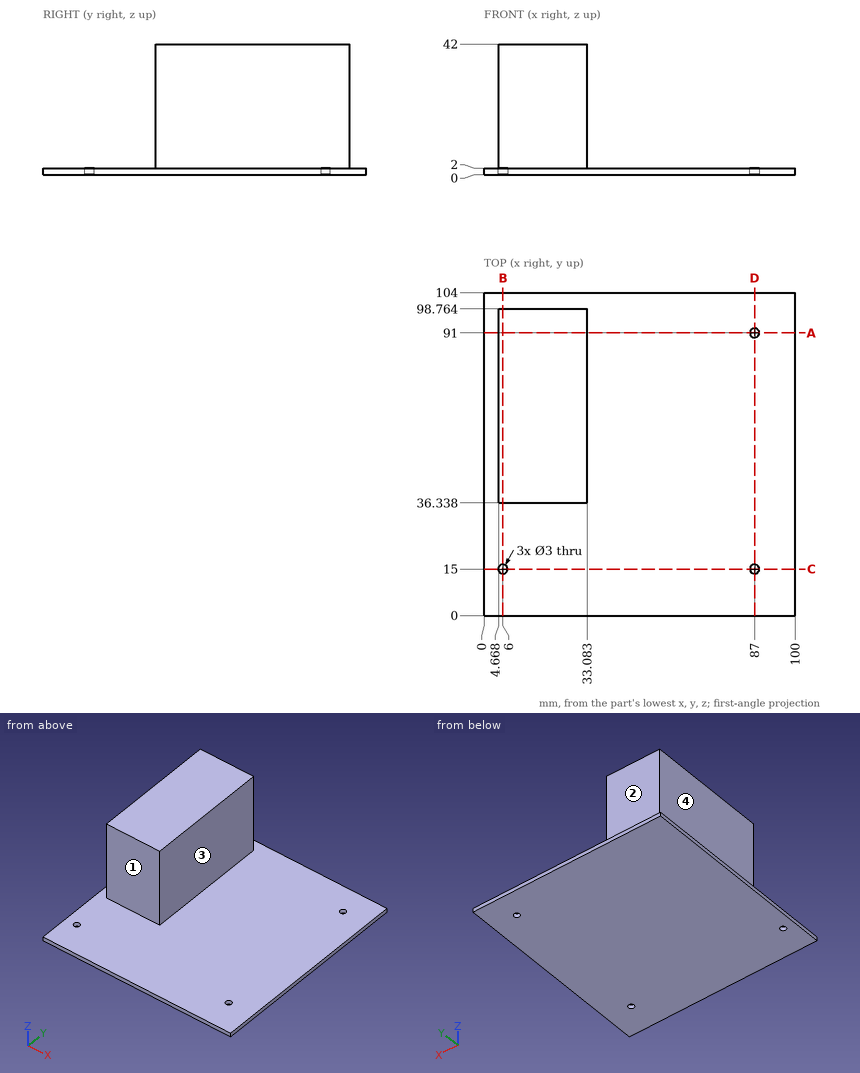
Answer from the drawing. Dimensions are ordinates in mm from the lowest x, y and z of the part. A direction names the side the tool comes from. Coordinates: 2 decimals unless noted, no trailing zeros. Loops run counter-clockwise (first coordinate to the right, second up) from the corner with the lowest first, then second, coordinate; pieces in that order, holes last. Notation, with made-up numbers: (-22, 71.5) -> (29, 71.5) arc R13 cw to (29, 91.5) -> close; hole circle Ø4 at (52.25, 84.25). An arc over 180 degrees is marked (long way). Return JSON: item names as keys, results as strings.
Item 1: For the marked faces 1, 2, 3 and 4, determine the directions among +Z, -Z, +X, -X, +Y, -Y from which every point of the face is accessible in a straight line to the end or side of a thin tool.
Answers:
{"face 1": "+Z, +X, -X, -Y", "face 2": "+Z, +X, -X, +Y", "face 3": "+Z, +X, +Y, -Y", "face 4": "+Z, -X, +Y, -Y"}
Item 2: Find section B-B (x = 6). Determine the outline of the cut face in (y, z).
Answers:
{"outline": "(0, 0) -> (13.5, 0) -> (13.5, 2) -> (0, 2) -> close; (16.5, 0) -> (104, 0) -> (104, 2) -> (98.76, 2) -> (98.76, 42) -> (36.34, 42) -> (36.34, 2) -> (16.5, 2) -> close"}
Item 3: Find section A-A (y = 91). Determine the outline of the cut face in (x, z), plus the area to 3 significant figures.
Answers:
{"outline": "(0, 0) -> (85.5, 0) -> (85.5, 2) -> (33.08, 2) -> (33.08, 42) -> (4.67, 42) -> (4.67, 2) -> (0, 2) -> close; (88.5, 0) -> (100, 0) -> (100, 2) -> (88.5, 2) -> close", "area": "1,330 mm2"}
Item 4: Find section C-C (y = 15). Determine the outline of the cut face in (x, z), plus the area to 3 significant figures.
Answers:
{"outline": "(0, 0) -> (4.5, 0) -> (4.5, 2) -> (0, 2) -> close; (7.5, 0) -> (85.5, 0) -> (85.5, 2) -> (7.5, 2) -> close; (88.5, 0) -> (100, 0) -> (100, 2) -> (88.5, 2) -> close", "area": "188 mm2"}
Item 5: Flat-ended cylindrical pins translate along their axes: P1, Ø5, axis at x = 87, y = 15, coming from the -Z side; P2, Ø12, axis at y = 44.5, z = 22.5, coming from the +X side; P3, Ø8, axis at x = 20.5, z = 9.5, coming from the -Y side; P4, Ø14, axis at x = 24, z = 16, coming from the +Y side. Find the tip coordinate at first contact, or state that the pin passes through.
Answers:
{"P1": "stops at z = 0", "P2": "stops at x = 33.08", "P3": "stops at y = 36.34", "P4": "stops at y = 98.76"}
Item 6: Find the intervals of material crossed by probe 1 along Z at (x, y) = (47.5, 89.5); probe 2 along X at (y, z) = (91, 0.65); probe 3 along X at (y, z) = (64.5, 22), in increasing order.
Answers:
{"probe 1": "z = 0 to 2", "probe 2": "x = 0 to 85.5, 88.5 to 100", "probe 3": "x = 4.67 to 33.08"}
Item 7: Find section D-D (x = 87). Determine the outline of the cut face in (y, z), plus the area to 3 significant figures.
Answers:
{"outline": "(0, 0) -> (13.5, 0) -> (13.5, 2) -> (0, 2) -> close; (16.5, 0) -> (89.5, 0) -> (89.5, 2) -> (16.5, 2) -> close; (92.5, 0) -> (104, 0) -> (104, 2) -> (92.5, 2) -> close", "area": "196 mm2"}
